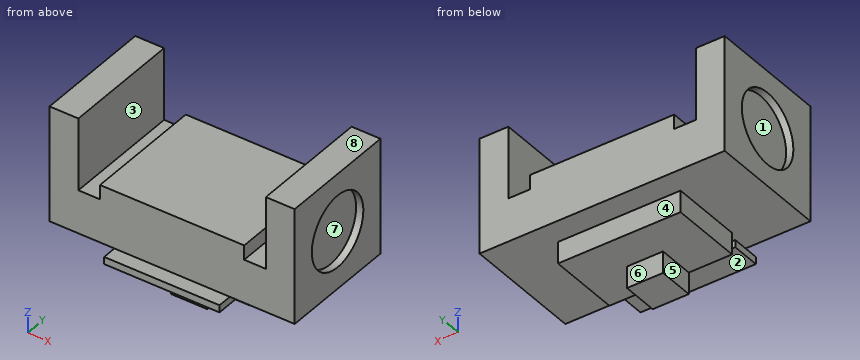
from build123d import *

# Parameters (mm, degrees)
SKETCH1_W           = 130
SKETCH1_H           = 83.238396624
BOSS_EXTRUDE1_DEPTH = 30
SKETCH2_W           = 100
SKETCH2_H           = 83.238396624
BOSS_EXTRUDE2_DEPTH = 10
SKETCH3_W           = 80
SKETCH3_H           = 83.238396624
BOSS_EXTRUDE3_DEPTH = 20
SKETCH4_R           = 25
CUT_EXTRUDE1_DEPTH  = 5
SKETCH5_W           = 80
SKETCH5_H           = 83.238396624
BOSS_EXTRUDE4_DEPTH = 20
CUT_EXTRUDE2_START  = -5
SKETCH6_R           = 25
CUT_EXTRUDE2_DEPTH  = 5
SKETCH7_W           = 80
SKETCH7_H           = 20
BOSS_EXTRUDE5_DEPTH = 5
SKETCH8_W           = 85
SKETCH8_H           = 50
BOSS_EXTRUDE6_DEPTH = 30
SKETCH9_W           = 85
SKETCH9_H           = 25
CUT_EXTRUDE3_DEPTH  = 15
SKETCH10_W          = 30
SKETCH10_H          = 15
CUT_EXTRUDE4_DEPTH  = 128.630488655


with BuildPart() as part:
    # Sketch1 → Boss-Extrude1 (new body)
    with BuildSketch(Plane.XY):
        Rectangle(SKETCH1_W, SKETCH1_H)
    extrude(amount=BOSS_EXTRUDE1_DEPTH)

    # Sketch2 → Boss-Extrude2 (add)
    with BuildSketch(Plane.XY.offset(30)):
        Rectangle(SKETCH2_W, SKETCH2_H)
    extrude(amount=BOSS_EXTRUDE2_DEPTH)

    # Sketch3 → Boss-Extrude3 (add)
    with BuildSketch(Plane.ZY.offset(65)):
        with Locations((40, 0)):
            Rectangle(SKETCH3_W, SKETCH3_H)
    extrude(amount=BOSS_EXTRUDE3_DEPTH)

    # Sketch4 → Cut-Extrude1 (cut)
    with BuildSketch(Plane.ZY.offset(85)):
        with Locations((40, 0)):
            Circle(SKETCH4_R)
    extrude(amount=-CUT_EXTRUDE1_DEPTH, mode=Mode.SUBTRACT)

    # Sketch5 → Boss-Extrude4 (add)
    with BuildSketch(Plane(origin=(65, 0, 0), x_dir=(0, 0, -1), z_dir=(1, 0, 0))):
        with Locations((-40, 0)):
            Rectangle(SKETCH5_W, SKETCH5_H)
    extrude(amount=BOSS_EXTRUDE4_DEPTH)

    # Sketch6 → Cut-Extrude2 (cut)
    with BuildSketch(Plane(origin=(85, 0, 0), x_dir=(0, 0, -1), z_dir=(1, 0, 0)).offset(CUT_EXTRUDE2_START)):
        with Locations(Location((-40, 0, 0), (0, 0, 180))):
            Circle(SKETCH6_R)
    extrude(amount=CUT_EXTRUDE2_DEPTH, mode=Mode.SUBTRACT)

    # Sketch7 → Boss-Extrude5 (add)
    with BuildSketch(Plane(origin=(0, 0, 0), x_dir=(-1, 0, 0), z_dir=(0, 0, -1))):
        with Locations((0, -41.619198312)):
            Rectangle(SKETCH7_W, SKETCH7_H)
    extrude(amount=BOSS_EXTRUDE5_DEPTH)

    # Sketch8 → Boss-Extrude6 (add)
    with BuildSketch(Plane(origin=(0, 0, 0), x_dir=(-1, 0, 0), z_dir=(0, 0, -1))):
        Rectangle(SKETCH8_W, SKETCH8_H)
    extrude(amount=BOSS_EXTRUDE6_DEPTH)

    # Sketch9 → Cut-Extrude3 (cut)
    with BuildSketch(Plane(origin=(0, 0, -30), x_dir=(-1, 0, 0), z_dir=(0, 0, -1))):
        with Locations((0, 12.5)):
            Rectangle(SKETCH9_W, SKETCH9_H)
    extrude(amount=-CUT_EXTRUDE3_DEPTH, mode=Mode.SUBTRACT)

    # Sketch10 → Cut-Extrude4 (cut, through all)
    with BuildSketch(Plane(origin=(0, 0, 0), x_dir=(1, 0, 0), z_dir=(0, 1, 0))):
        with Locations((-27.5, 22.5)):
            Rectangle(SKETCH10_W, SKETCH10_H)
        with Locations((27.5, 22.5)):
            Rectangle(SKETCH10_W, SKETCH10_H)
    extrude(amount=-CUT_EXTRUDE4_DEPTH, mode=Mode.SUBTRACT)


solid = part.part
Geometry: final body of the model. Coordinates: model frame, mm. Face numbers are marked on the shaded views. A direction names the side the tool comes from. Give positions to 0.01 mm unless a question says otherwise; leave off trailing zeros. Write each loop counter-clockwise with the first axis right and the second up, starting at its lowest first coordinate (ties: lowest second). Pieces come first, ordered by that corner, then holes.
(1) Cut plane A-A, the plane z = 45. Return loops of the section in (x, y).
(2) First-contact query: P1, Ø25, axis at y = 2, z = 49, coming from the -X side; P2, Ø4, axis at x = 60.5, y = -17.5, coming from the -Z side; P3, Ø11, axis at y = -17.5, z = 36, coming from the +X side; P4, Ø5, axis at y = -29, z = -3.5, coming from the -X side. Flat tips, straight axial feed; report the tip coordinate or a pass-through.
(3) Cut plane D-D, the plane y = -39.5. Return loops of the section in (x, z).
(4) Cut plane C-C, the plane x = -20.5. Return loops of the section in (y, z), then the cut area to 3 significant figures.
(5) Access query for the marked faces 1, 2, 3, 4 and 5. Directions: +Z, -Z, +X, -X, +Y, -Y. A direction counts if a zero-diameter tool reaches every point of the face in a straight line with its end or side. Return the directions, or none.
(6) Ray query, line 1 (X direction, y = 14, z = 32.5); line 2 (Y direction, x = -83.35, z = 40); line 3 (X direction, y = -25, z = 51). Return the intervals inside material, ascending.
(7) Mould query, pull axis Z, two halves, no side actions, for the marked faces 6, 7 and 8. Classes: released by +Z, released by -Z, zero draft, split by the parting line, or undercut.
(8) Cut plane B-B, the plane y = -28.5. Return loops of the section in (x, z).
Values follow:
1. outline: (-85, -41.62) - (-65, -41.62) - (-65, 41.62) - (-85, 41.62) - (-85, 24.49) - (-80, 24.49) - (-80, -24.49) - (-85, -24.49) - close; (65, -41.62) - (85, -41.62) - (85, -24.49) - (80, -24.49) - (80, 24.49) - (85, 24.49) - (85, 41.62) - (65, 41.62) - close
2. P1: stops at x = -80
2. P2: stops at z = 0
2. P3: stops at x = 80
2. P4: passes through
3. outline: (-85, 0) - (-40, 0) - (-40, -5) - (40, -5) - (40, 0) - (85, 0) - (85, 80) - (65, 80) - (65, 30) - (50, 30) - (50, 40) - (-50, 40) - (-50, 30) - (-65, 30) - (-65, 80) - (-85, 80) - close
4. outline: (-51.62, -5) - (-31.62, -5) - (-31.62, 0) - (-25, 0) - (-25, -15) - (25, -15) - (25, 0) - (41.62, 0) - (41.62, 40) - (-41.62, 40) - (-41.62, 0) - (-51.62, 0) - close
4. area: 4,180 mm2
5. face 1: -X
5. face 2: -Z, +X, -X, -Y
5. face 3: +Z, +Y, -Y
5. face 4: -Z, +X, -X, +Y
5. face 5: -Z, -X, +Y, -Y
6. line 1: x = -80 to -65, -50 to 50, 65 to 80
6. line 2: y = -41.62 to -25, 25 to 41.62
6. line 3: x = -85 to -65, 65 to 85
7. face 6: zero draft
7. face 7: undercut
7. face 8: released by +Z
8. outline: (-85, 0) - (85, 0) - (85, 80) - (65, 80) - (65, 30) - (50, 30) - (50, 40) - (-50, 40) - (-50, 30) - (-65, 30) - (-65, 80) - (-85, 80) - close
